Read the model definition and answer for the solid it produces. Units are mm, in the model's axes. Face numbers are marked on the shaded views. A direction names the side the tool comes from. Coordinates: 2 decimals unless noted, no trailing zeros. Answer as a JSON object with one key per item and string values. Group by question number.
1) Given pin 1 (2 mm diameter, centred on x = 59.5, y = 2.5, fed in from -Z); pin 2 (10 mm diameter, centred on x = 28.5, z = -9.5, fed in from +Y); pin 3 (1.5 mm diameter, centred on y = -13.5, z = 9, fed in from -X); pin 4 (5.5 mm diameter, centred on y = 66.42, z = -11.43, fed in from -X), each flat-ended and moving along its own axis, determine where each tip first touches the part or whether it passes through.
2) Section A-A on y = 66 is taken. Count the separate pieces of the cut face and the enclosed holes in it, and give its area (3 significant figures).
3) A tool of negligible diameter and unlimited length cuts with its end or side. For the marked faces 1, 2 and 3, from which of +Z, -Z, +X, -X, +Y, -Y can it reach the whole face along a straight path? Write none if from no direction.
4) Consider L1, parallel to Y at x = 9, z = 13.97; L2, parallel to Y at x = 9, z = 12.5; L3, parallel to Z at x = 51, y = 23.5. Determine where each line is inside the solid, lowest interval first.
5) Determine the mould class of the marked faces 4, 5 and 6 for opening direction Y: released by +Y, released by -Y, zero draft, split by the parting line, or undercut.
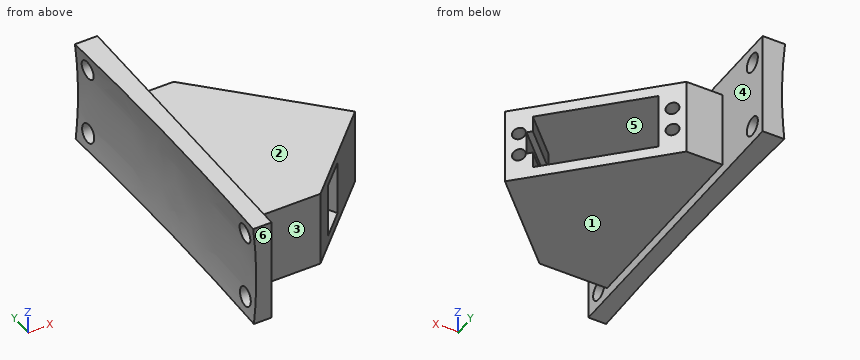
from build123d import *

# Parameters (mm, degrees)
SKETCH1_W               = 15.24
SKETCH1_H               = 47.25
BOSS_EXTRUDE1_DEPTH     = 29
BOSS_EXTRUDE2_DEPTH     = 15.24
BOSS_EXTRUDE3_START     = 6.35
BOSS_EXTRUDE3_DEPTH     = 27.94
CUT_EXTRUDE4_DEPTH      = 90.856122335
CUT_EXTRUDE4_DEPTH_BACK = 90.856122335
BOSS_EXTRUDE4_START     = 12.7
SKETCH15_W              = 12.73404056
SKETCH15_H              = 107.95
BOSS_EXTRUDE4_DEPTH     = 38.1
SKETCH17_R              = 3.429
CUT_EXTRUDE6_DEPTH      = 95.762638832
BOSS_EXTRUDE9_DEPTH     = 6.35
BOSS_EXTRUDE10_DEPTH    = 6.35
SKETCH12_W              = 20.20062
SKETCH12_H              = 40.64
CUT_EXTRUDE8_DEPTH      = 38.1
SKETCH21_W              = 27.94
SKETCH21_H              = 50.342193805
CUT_EXTRUDE9_DEPTH      = 8
SKETCH22_W              = 27.94
SKETCH22_H              = 8
CUT_EXTRUDE10_DEPTH     = 2.54
BOSS_EXTRUDE11_DEPTH    = 13.97
SKETCH24_W              = 11.491520074
SKETCH24_H              = 20.20062
CUT_EXTRUDE11_DEPTH     = 112.502999945
SKETCH25_R              = 2.249999945
CUT_EXTRUDE12_DEPTH     = 18
CUT_EXTRUDE13_REACH     = 83.705
SKETCH26_W              = 8.500000018
SKETCH26_H              = 2.032


with BuildPart() as part:
    # Sketch1 → Boss-Extrude1 (new body)
    with BuildSketch(Plane(origin=(0, 0, 0), x_dir=(0, 0, -1), z_dir=(1, 0, 0))):
        Rectangle(SKETCH1_W, SKETCH1_H)
    extrude(amount=BOSS_EXTRUDE1_DEPTH)

    # Sketch8 → Cut-Revolve1 (revolve, cut)
    with BuildSketch(Plane(origin=(0, 0, 0), x_dir=(1, 0, 0), z_dir=(0, 1, 0))):
        with BuildLine():
            Line((-1363.98, 509.27), (-1363.98, -509.27))
            add(Edge.make_bspline(
                [(-1363.98, -509.27), (8.89, -509.27), (8.89, 0), (8.89, 509.27), (-1363.98, 509.27)],
                knots=[4.71238898, 4.71238898, 4.71238898, 6.283185307, 6.283185307, 7.853981634, 7.853981634, 7.853981634], degree=2, weights=[1, 0.707106781, 1, 0.707106781, 1]))
        make_face()
    revolve(axis=Axis((-1363.98, 0, -509.27), (0, 0, 1)), mode=Mode.SUBTRACT)

    # Sketch9 → Boss-Extrude2 (add)
    with BuildSketch(Plane.XY.offset(7.62)):
        Polygon((29, -23.625), (57.293684645, -23.625), (29, 23.625), align=None)
    extrude(amount=-BOSS_EXTRUDE2_DEPTH)

    # Sketch11 → Boss-Extrude3 (add)
    with BuildSketch(Plane(origin=(0, 0, -7.62), x_dir=(-1, 0, 0), z_dir=(0, 0, -1)).offset(BOSS_EXTRUDE3_START)):
        Polygon((-8.532999942, 23.625), (-35.473768305, 50.565768363), (-71.071074924, 14.968461744), (-48.544371121, -9.013786608), (-28.889356272, 23.625), align=None)
    extrude(amount=-BOSS_EXTRUDE3_DEPTH)

    # Sketch13 → Cut-Extrude4 (cut, two sides: drawn at the far end of the back side and taken through both)
    with BuildSketch(Plane(origin=(0, 0, -7.62), x_dir=(-1, 0, 0), z_dir=(0, 0, -1)).offset(-CUT_EXTRUDE4_DEPTH_BACK)):
        Polygon((-61.672265147, 5.569651967), (-8.532999942, -23.625), (-25.02523354, -53.6436889), (-79.417056311, -23.760883228), align=None)
    extrude(amount=CUT_EXTRUDE4_DEPTH + CUT_EXTRUDE4_DEPTH_BACK, mode=Mode.SUBTRACT)

    # Sketch15 → Boss-Extrude4 (add)
    with BuildSketch(Plane.XY.offset(7.62).offset(BOSS_EXTRUDE4_START)):
        with Locations((7.499979662, 18.790026662)):
            Rectangle(SKETCH15_W, SKETCH15_H)
    extrude(amount=-BOSS_EXTRUDE4_DEPTH)

    # Sketch16 → Cut-Revolve2 (revolve, cut)
    with BuildSketch(Plane(origin=(0, 0, 0), x_dir=(1, 0, 0), z_dir=(0, 1, 0))):
        with BuildLine():
            Line((-1364.099005706, 509.27), (-1364.099005706, -509.27))
            add(Edge.make_bspline(
                [(-1364.099005706, -509.27), (8.770994294, -509.27), (8.770994294, 0), (8.770994294, 509.27), (-1364.099005706, 509.27)],
                knots=[4.71238898, 4.71238898, 4.71238898, 6.283185307, 6.283185307, 7.853981634, 7.853981634, 7.853981634], degree=2, weights=[1, 0.707106781, 1, 0.707106781, 1]))
        make_face()
    revolve(axis=Axis((-1364.099005706, 0, -509.27), (0, 0, 1)), mode=Mode.SUBTRACT)

    # Sketch17 → Cut-Extrude6 (cut, through all)
    with BuildSketch(Plane(origin=(13.866999942, 0, 0), x_dir=(0, 0, -1), z_dir=(1, 0, 0))):
        with Locations(Location((-13.97, -28.834973338, 0), (0, 0, 90))):
            Circle(SKETCH17_R)
        with Locations(Location((-13.97, 66.415026662, 0), (0, 0, 90))):
            Circle(SKETCH17_R)
        with Locations(Location((11.43, 66.415026662, 0), (0, 0, 90))):
            Circle(SKETCH17_R)
        with Locations(Location((11.43, -28.834973338, 0), (0, 0, 90))):
            Circle(SKETCH17_R)
    extrude(amount=-CUT_EXTRUDE6_DEPTH, mode=Mode.SUBTRACT)

    # Sketch19 → Boss-Extrude9 (add)
    with BuildSketch(Plane.XY.offset(7.62)):
        Polygon((13.866999942, 23.625), (13.866999942, -20.694506456), (45.209055073, -3.475216955), (28.889356272, 23.625), align=None)
    extrude(amount=BOSS_EXTRUDE9_DEPTH)

    # Sketch20 → Boss-Extrude10 (add)
    with BuildSketch(Plane(origin=(0, 0, -7.62), x_dir=(-1, 0, 0), z_dir=(0, 0, -1))):
        Polygon((-45.209055073, -3.475216955), (-13.866999942, -20.694506456), (-13.866999942, 23.625), (-28.889356272, 23.625), align=None)
    extrude(amount=BOSS_EXTRUDE10_DEPTH)

    # Sketch12 → Cut-Extrude8 (cut)
    with BuildSketch(Plane(origin=(43.019768334, 43.019768334, 0), x_dir=(0, 0, -1), z_dir=(0.7071067811865476, 0.7071067811865476, 0))):
        with Locations((0, -14.49944132)):
            Rectangle(SKETCH12_W, SKETCH12_H)
    extrude(amount=-CUT_EXTRUDE8_DEPTH, mode=Mode.SUBTRACT)

    # Sketch21 → Cut-Extrude9 (cut)
    with BuildSketch(Plane(origin=(43.019768334, 43.019768334, 0), x_dir=(0, 0, -1), z_dir=(0.7071067811865477, 0.7071067811865475, 0))):
        with Locations((0, -14.49944132)):
            Rectangle(SKETCH21_W, SKETCH21_H)
    extrude(amount=-CUT_EXTRUDE9_DEPTH, mode=Mode.SUBTRACT)

    # Sketch22 → Cut-Extrude10 (cut)
    with BuildSketch(Plane(origin=(28.05130659, -28.05130659, 0), x_dir=(0, 0, 1), z_dir=(-0.7071067811865476, 0.7071067811865476, 0))):
        with Locations((0, 56.839139829)):
            Rectangle(SKETCH22_W, SKETCH22_H)
    extrude(amount=-CUT_EXTRUDE10_DEPTH, mode=Mode.SUBTRACT)

    # Sketch23 → Boss-Extrude11 (add, symmetric)
    with BuildSketch(Plane.XY):
        Polygon((29.816914056, 44.908914114), (26.883196541, 47.842631629), (13.866999942, 47.842631629), (13.866999942, 28.959), align=None)
        Polygon((65.591257632, 9.134570538), (13.866999942, -20.694506456), (13.866999942, -23.674292513), (38.295755697, -23.674292513), (68.34793819, 6.37788998), align=None)
    extrude(amount=BOSS_EXTRUDE11_DEPTH, both=True)

    # Sketch24 → Cut-Extrude11 (cut, through all)
    with BuildSketch(Plane(origin=(12.416727049, -21.530870355, 0), x_dir=(0.8662714122168664, 0.49957365860881403, 0), z_dir=(-0.49957365860881403, 0.8662714122168664, 0))):
        with Locations((35.963054904, 0)):
            Rectangle(SKETCH24_W, SKETCH24_H)
    extrude(amount=-CUT_EXTRUDE11_DEPTH, mode=Mode.SUBTRACT)

    # Sketch25 → Cut-Extrude12 (cut)
    with BuildSketch(Plane(origin=(37.362914085, 37.362914085, 0), x_dir=(0, 0, -1), z_dir=(0.7071067811865476, 0.7071067811865475, 0))):
        with Locations(Location((-4.250000009, 10.32055868, 0), (0, 0, 90))):
            Circle(SKETCH25_R)
        with Locations(Location((4.250000009, 10.32055868, 0), (0, 0, 90))):
            Circle(SKETCH25_R)
        with Locations(Location((-4.250000009, -39.31944132, 0), (0, 0, 90))):
            Circle(SKETCH25_R)
        with Locations(Location((4.250000009, -39.31944132, 0), (0, 0, 90))):
            Circle(SKETCH25_R)
    extrude(amount=-CUT_EXTRUDE12_DEPTH, mode=Mode.SUBTRACT)

    # Cut-Extrude13: up to this plane
    cut_extrude13_end = Plane(origin=(68.733790735, -35.697044307, 10.10031), z_dir=(0.8662714122168665, 0.49957365860881403, -3.0669196206838748e-15))
    # Sketch26 → Cut-Extrude13 (cut, up to the surface)
    with BuildSketch(Plane(origin=(37.362914085, 37.362914085, 0), x_dir=(0, 0, -1), z_dir=(0.7071067811865476, 0.7071067811865475, 0)), mode=Mode.PRIVATE) as cut_extrude13_sk1:
        with Locations((0, -35.83544132)):
            Rectangle(SKETCH26_W, SKETCH26_H)
    cut_extrude13_tool1 = split(extrude(cut_extrude13_sk1.sketch, amount=-CUT_EXTRUDE13_REACH, mode=Mode.PRIVATE), bisect_by=cut_extrude13_end, keep=Keep.BOTH, mode=Mode.PRIVATE)
    add(cut_extrude13_tool1.solids().sort_by_distance((62.702398, 12.023431, 0))[0], mode=Mode.SUBTRACT)


solid = part.part
Worked answers:
{
 "1": {"pin 1": "stops at z = -13.97", "pin 2": "stops at y = 47.84", "pin 3": "stops at x = 8.45", "pin 4": "passes through"},
 "2": {"separate pieces": "3", "enclosed holes": "0", "area": "170 mm²"},
 "3": {"face 1": "-Z, +X, +Y, -Y", "face 2": "+Z, +X, +Y, -Y", "face 3": "+Z, -Z, +X, -Y"},
 "4": {"L1": "y = -35.18 to -32.26, -25.41 to 62.99, 69.84 to 72.77", "L2": "y = -35.18 to -31.93, -25.74 to 63.32, 69.51 to 72.77", "L3": "z = -13.97 to -10.1, 10.1 to 13.97"},
 "5": {"face 4": "zero draft", "face 5": "undercut", "face 6": "released by -Y"}
}
